Part print with two shaded views. Sizes in mm from the minimum x, y, z corner. A direction names the side the tool comes from. Coordinates: 2 decimals unless noted, no trailing zeros. One line per question, with ' | ' between items. Start each with the question number.
1. Probe line 1 (X direction, y = 3.25, z = 20) (1 decimal); line 2 (Z direction, x = 36, y = 3.5); line 3 (Z direction, x = 12, y = 2.25) (1 decimal). List the from-to ranges inside material, lowest first.
2. Two-plate mould, pull along Z, no slides. Class the marked faces 1, 2, 3 and 4: +Z half, -Z half, draft (parallel to the pull), parting line (faces both ways), or undercut.
3. Flat gauge pins, fed straight in: P1, Ø1.9, axis at y = 4, z = 24.5, coming from the -X side; P2, Ø2, axis at x = 24.5, y = 5, coming from the +Z side; P3, Ø1.5, axis at x = 8.5, y = 3, coming from the +Z side. Where does each tip first touch, or does it go through?
4. Which spindle directions (+Z, -Z, +X, -X, +Y, -Y) get a long thin tool onto all of the face, cutting with end or side? Do the marked faces 5, 6 and 7. Say none if no direction does.
5. Band-saw the part on A-A, the plane y = 5.25. Give the number of separate pieces and of enclosed holes in the cut face, then the cut area to 3 significant figures.
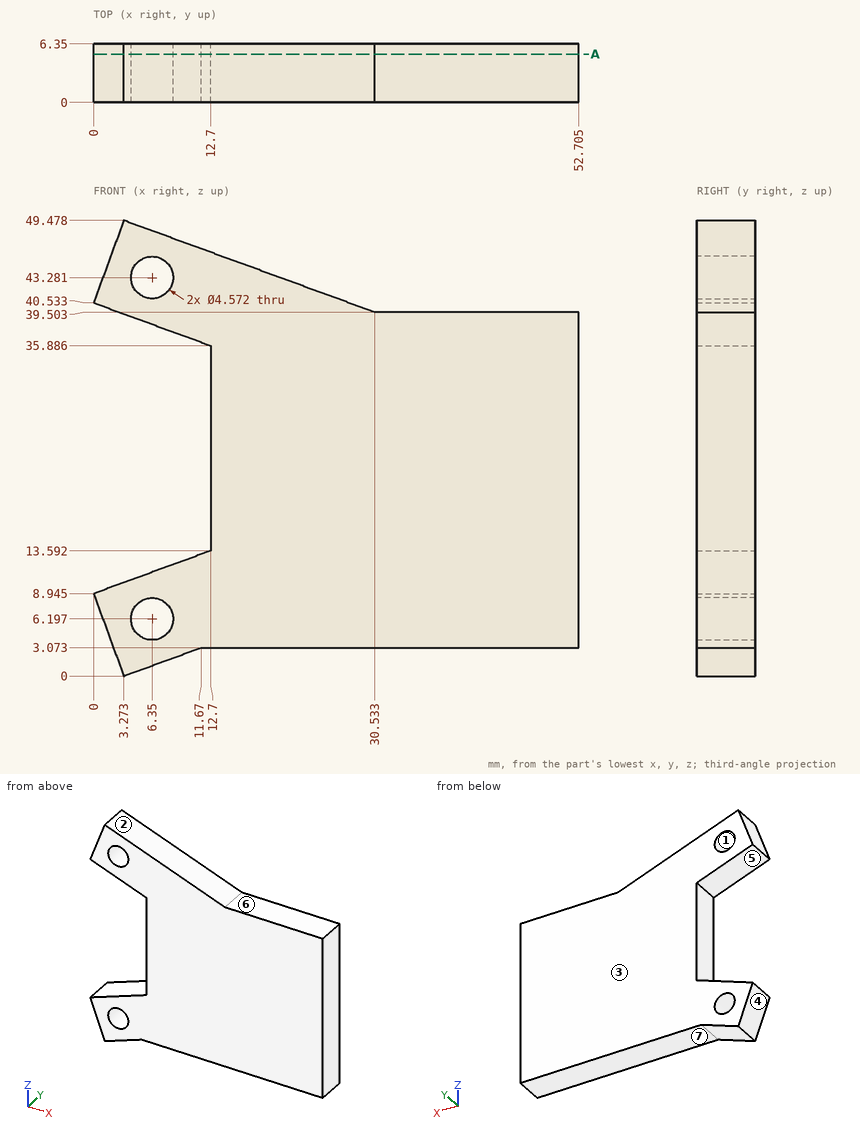
Filled in:
1) line 1: x = 12.7 to 52.7 | line 2: z = 3.07 to 39.5 | line 3: z = 3.1 to 13.3, 36.1 to 46.3
2) face 1: undercut | face 2: +Z half | face 3: draft | face 4: -Z half
3) P1: stops at x = 12.7 | P2: stops at z = 42.08 | P3: stops at z = 47.84
4) face 5: -X, +Y, -Y | face 6: +Z, +X, +Y, -Y | face 7: -Z, +X, +Y, -Y
5) separate pieces: 1 | enclosed holes: 2 | area: 1,710 mm²
